Read the model definition and answer for the solid it produces. Units are mm, in the model's axes. Face numbers are marked on the shaded views. A direction names the side the tool comes from. Coordinates: 2 decimals unless noted, no trailing zeros. Order: outer loops, then holes, each group sorted by start corner. A loop starts at its lowest first (then second) coordinate and runs counter-clockwise, first axis right, second up. Notation, with made-up numbers: M 87.25,68 L 111.25,68 A18 ccw 111.25,97 Z; hole C -32.75,4.5 d10. An arc over 180 degrees is marked long. Use a Markdown table: item, result. Add a question column.
1) Find section D-D on y = 3.5. Write down the section's boundary in (x, z).
2) Find section C-C on z = 17.75. Write down the section's boundary in (x, y).
3) Find section B-B on x = 16.65. Write down the section's boundary in (y, z).
4) Find section A-A on z = 10. Write down the section's boundary in (x, y), plus the area to 3 significant figures.
5) Find the intervals of material crossed by probe 1 along Y at (x, z) = (0, 6.5); probe 2 along Z at (x, y) = (16.65, -16.3); probe 3 along Y at (x, z) = (12.5, 16), in increasing order. Write a range as [from, to].
6) For the marked faces 1, 2 and 3, determine the directions among +Z, -Z, +X, -X, +Y, -Y from which every point of the face is accessible in a straight line to the end or side of a thin tool.
7) The mould has two halves that part along Z. Classify the marked faces 4, 5 and 6: released by +Z, released by -Z, zero draft, split by the parting line, or undercut.
8) Each of these flat-tipped pins is pushed along its axis until it touches: pin 1 Ø6 at (y, z) = (-4.5, 10.5) entering from +X; pin 2 Ø11.5 at (x, y) = (0, 0) entering from -Z; pin 3 Ø7 at (x, z) = (17.5, 9.5) entering from +Y; pin 4 Ø1.5 at (x, z) = (7.5, 8.5) entering from +Y. Where does it stop, or does it pass through?
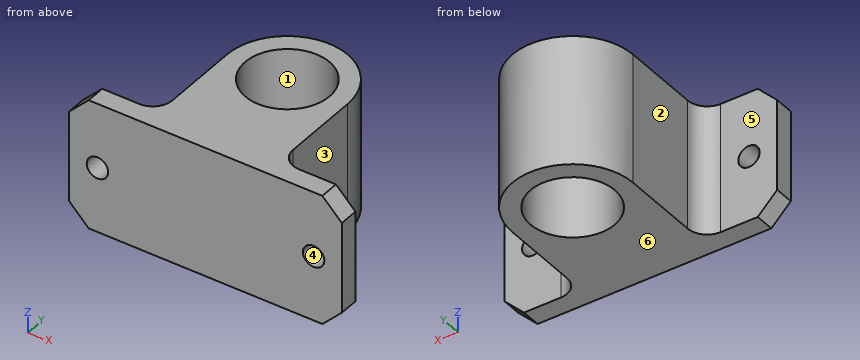
from build123d import *

# Parameters (mm, degrees)
SKETCH1_R           = 6.5
BOSS_EXTRUDE1_DEPTH = 20
CHAMFER1_SIZE       = 3
SKETCH2_R           = 1.65
CUT_EXTRUDE1_DEPTH  = 20


with BuildPart() as part:
    # Sketch1 → Boss-Extrude1 (new body)
    with BuildSketch(Plane.XY):
        with BuildLine():
            Line((-21, -18.072367328), (21, -18.072367328))
            Line((21, -18.072367328), (21, -15.072367328))
            Line((21, -15.072367328), (12.3, -15.072367328))
            ThreePointArc((12.3, -15.072367328), (10.178679656, -14.193687672), (9.3, -12.072367328))
            Line((9.3, -12.072367328), (9.3, 0))
            ThreePointArc((9.3, 0), (0, 9.3), (-9.3, 0))
            Line((-9.3, 0), (-9.3, -12.072367328))
            ThreePointArc((-9.3, -12.072367328), (-10.178679656, -14.193687672), (-12.3, -15.072367328))
            Line((-12.3, -15.072367328), (-21, -15.072367328))
            Line((-21, -15.072367328), (-21, -18.072367328))
        make_face()
        Circle(SKETCH1_R, mode=Mode.SUBTRACT)
    extrude(amount=BOSS_EXTRUDE1_DEPTH)

    # Chamfer1
    chamfer1_edges = [part.edges().sort_by_distance(p)[0] for p in [
        (21, -16.572367328, 20),
        (21, -16.572367328, 0),
        (-21, -16.572367328, 0),
        (-21, -16.572367328, 20),
    ]]
    chamfer(chamfer1_edges, length=CHAMFER1_SIZE)

    # Sketch2 → Cut-Extrude1 (cut)
    with BuildSketch(Plane(origin=(0, -15.072367328, 0), x_dir=(1, 0, 0), z_dir=(0, 1, 0))):
        with Locations(Location((16.65, -10, 0), (0, 0, 180))):
            Circle(SKETCH2_R)
        with Locations(Location((-16.65, -10, 0), (0, 0, 180))):
            Circle(SKETCH2_R)
    extrude(amount=-CUT_EXTRUDE1_DEPTH, mode=Mode.SUBTRACT)


solid = part.part
Check result:
| question | item | result |
|---|---|---|
| 1 | outline | M -8.62,0 L -5.48,0 L -5.48,20 L -8.62,20 Z; M 5.48,0 L 8.62,0 L 8.62,20 L 5.48,20 Z |
| 2 | outline | M -20.25,-18.07 L 20.25,-18.07 L 20.25,-15.07 L 12.3,-15.07 A3 cw 9.3,-12.07 L 9.3,0 A9.3 ccw -9.3,0 L -9.3,-12.07 A3 cw -12.3,-15.07 L -20.25,-15.07 Z; hole C 0,0 d13 |
| 3 | outline | M -18.07,0 L -15.07,0 L -15.07,8.35 L -18.07,8.35 Z; M -18.07,11.65 L -15.07,11.65 L -15.07,20 L -18.07,20 Z |
| 4 | outline | M -21,-18.07 L -18.3,-18.07 L -18.3,-15.07 L -21,-15.07 Z; M -15,-18.07 L 15,-18.07 L 15,-15.07 L 12.3,-15.07 A3 cw 9.3,-12.07 L 9.3,0 A9.3 ccw -9.3,0 L -9.3,-12.07 A3 cw -12.3,-15.07 L -15,-15.07 Z; M 18.3,-18.07 L 21,-18.07 L 21,-15.07 L 18.3,-15.07 Z; hole C 0,0 d13 |
| 4 | area | 394 mm2 |
| 5 | probe 1 | y = [-18.07, -6.5], [6.5, 9.3] |
| 5 | probe 2 | z = [0, 8.35], [11.65, 20] |
| 5 | probe 3 | y = [-18.07, -15.07] |
| 6 | face 1 | +Z, -Z |
| 6 | face 2 | +Z, -Z, -X, +Y |
| 6 | face 3 | +Z, -Z, +X, +Y |
| 7 | face 4 | undercut |
| 7 | face 5 | zero draft |
| 7 | face 6 | released by -Z |
| 8 | pin 1 | stops at x = 9.3 |
| 8 | pin 2 | passes through |
| 8 | pin 3 | stops at y = -15.07 |
| 8 | pin 4 | stops at y = 6.4 |
